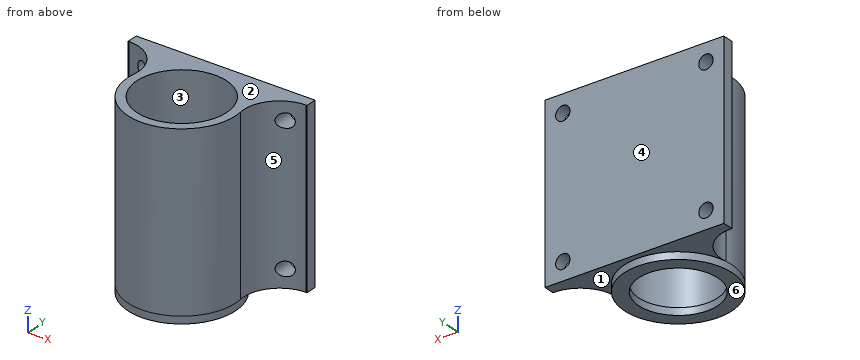
from build123d import *

# Parameters (mm, degrees)
SKETCH1_R           = 12.5
BOSS_EXTRUDE1_DEPTH = 48
BOSS_EXTRUDE3_START = 2
SKETCH3_R           = 15
SKETCH3_R_2         = 11
BOSS_EXTRUDE3_DEPTH = 2
SKETCH4_R           = 2
CUT_EXTRUDE1_DEPTH  = 63.623877738


with BuildPart() as part:
    # Sketch1 → Boss-Extrude1 (new body)
    with BuildSketch(Plane.XY):
        with BuildLine():
            Line((24.754908454, 13.492063492), (25, 13.492063492))
            Line((25, 13.492063492), (25, 16.507936508))
            Line((25, 16.507936508), (-25, 16.507936508))
            Line((-25, 16.507936508), (-25, 13.492063492))
            Line((-25, 13.492063492), (-24.754908454, 13.492063492))
            ThreePointArc((-24.754908454, 13.492063492), (-17.206125308, 10.050712211), (-14.852945072, 2.095238095))
            ThreePointArc((-14.852945072, 2.095238095), (0, -15), (14.852945072, 2.095238095))
            ThreePointArc((14.852945072, 2.095238095), (17.206125308, 10.050712211), (24.754908454, 13.492063492))
        make_face()
        Circle(SKETCH1_R, mode=Mode.SUBTRACT)
    extrude(amount=BOSS_EXTRUDE1_DEPTH)

    # Sketch3 → Boss-Extrude3 (add)
    with BuildSketch(Plane(origin=(0, 0, 0), x_dir=(-1, 0, 0), z_dir=(0, 0, -1)).offset(BOSS_EXTRUDE3_START)):
        Circle(SKETCH3_R)
        Circle(SKETCH3_R_2, mode=Mode.SUBTRACT)
    extrude(amount=-BOSS_EXTRUDE3_DEPTH)

    # Sketch4 → Cut-Extrude1 (cut, through all)
    with BuildSketch(Plane(origin=(0, 16.507936508, 0), x_dir=(1, 0, 0), z_dir=(0, 1, 0))):
        with Locations(Location((-20, -5, 0), (0, 0, 270))):
            Circle(SKETCH4_R)
        with Locations(Location((20, -5, 0), (0, 0, 270))):
            Circle(SKETCH4_R)
        with Locations(Location((20, -43, 0), (0, 0, 270))):
            Circle(SKETCH4_R)
        with Locations(Location((-20, -43, 0), (0, 0, 270))):
            Circle(SKETCH4_R)
    extrude(amount=-CUT_EXTRUDE1_DEPTH, mode=Mode.SUBTRACT)


solid = part.part
Verification items for the finished model (mm, model axes). Face numbers are marked on the shaded views. A direction names the side the tool comes from. Coordinates: 2 decimals unless noted, no trailing zeros. Order: outer loops, then holes, each group sorted by start corner. A loop starts at its lowest first (then second) coordinate and runs counter-clockwise, first axis right, second up.
Item 1: Release check for a two-part mould opening along Y. For the marked faces 4, 5 and 6 record: +Y half, -Y half, draft (parallel to the pull), parting line (faces both ways), or undercut.
Filled in:
face 4: +Y half
face 5: undercut
face 6: draft
Item 2: Depth check by flat-ended pin: pin 1 (4 mm diameter, centred on y = -5.5, z = 7.5, fed in from +X); pin 2 (4 mm diameter, centred on x = 6, z = 41.5, fed in from -Y); pin 3 (6 mm diameter, centred on y = 7, z = 35.5, fed in from +X). Enter the tip coordinate at first touch or a pass-through.
Filled in:
pin 1: stops at x = 14.59
pin 2: stops at y = -14.46
pin 3: stops at x = 17.16
Item 3: Section check D-D, the plane x = 20. Enter the section's corners in (y, z).
Filled in:
outline: (12.29, 0) - (16.51, 0) - (16.51, 3) - (12.29, 3) - close; (12.29, 7) - (16.51, 7) - (16.51, 41) - (12.29, 41) - close; (12.29, 45) - (16.51, 45) - (16.51, 48) - (12.29, 48) - close
Item 4: Material ranges on L1, parallel to X at y = 13.75, z = 43; L2, parallel to Y at x = 0, z = 20; L3, parallel to Y at x = -18, z = 1.5, recorded low to high.
Filled in:
L1: x = -25 to -22, -18 to 18, 22 to 25
L2: y = -15 to -12.5, 12.5 to 16.51
L3: y = 10.87 to 16.51
Item 5: Section check B-B, the plane z = 43. Enter the section's corners in (x, y).
Filled in:
outline: (-25, 13.49) - (-24.75, 13.49) arc R10 cw to (-22, 13.11) - (-22, 16.51) - (-25, 16.51) - close; (-18, 10.87) arc R10 cw to (-14.85, 2.1) arc R15 ccw (long way) to (14.85, 2.1) arc R10 cw to (18, 10.87) - (18, 16.51) - (-18, 16.51) - close; (22, 13.11) arc R10 cw to (24.75, 13.49) - (25, 13.49) - (25, 16.51) - (22, 16.51) - close; hole circle Ø25 at (0, 0)
Item 6: Section check A-A, the plane x = 0. Enter the section's corners in (y, z), then the cut area to 3 significant figures.
Filled in:
outline: (-15, -2) - (-11, -2) - (-11, 0) - (-12.5, 0) - (-12.5, 48) - (-15, 48) - close; (11, -2) - (15, -2) - (15, 0) - (16.51, 0) - (16.51, 48) - (12.5, 48) - (12.5, 0) - (11, 0) - close
area: 328 mm2
Item 7: Access from +Z, -Z, +X, -X, +Y, -Y to the whole of each face (thin tool, end or side, straight path). Record for the marked faces 1, 2 and 3.
Filled in:
face 1: -Z, +Y
face 2: +Z, +X, -X, +Y, -Y
face 3: +Z
Item 8: Section check C-C, the plane y = 1. Enter the section's corners in (x, z).
Filled in:
outline: (-14.97, -2) - (-10.95, -2) - (-10.95, 0) - (-12.46, 0) - (-12.46, 48) - (-14.97, 48) - close; (10.95, -2) - (14.97, -2) - (14.97, 48) - (12.46, 48) - (12.46, 0) - (10.95, 0) - close
